Here's how the part is built. I have some questions about the finished solid (model axes, mm). A direction names the side the tool comes from. Coordinates: 2 decimals unless noted, no trailing zeros. Write each loop counter-clockwise with the first axis right and the second up, starting at its lowest first coordinate (ties: lowest second). Pieces come first, ordered by that corner, then holes. Notation, with made-up numbers: (58.5, 62.25) -> (102.5, 62.25) arc R12 cw to (102.5, 75.25) -> close; hole circle Ø1 at (54.5, 87.25). An arc over 180 degrees is marked (long way). Put each result on its own line as item: value. Start each with the question number.
Item 1: I need wall thicknesses on line 1 (Y direction, x = -3.5, z = 9.5); line 2 (X direction, y = 45.5, z = -1); line 3 (Y direction, x = -2, z = 5.25). Which ranges of each line are inside material? Lowest first, please. Write a range as [from, to].
Item 2: I want a section at B-B, the plane x = 0. List the corners of the cut face in (y, z) for me, then the cut area to 3 significant figures.
Item 3: I want a section at A-A, the plane y = 42. List the corners of the cut face in (x, z) for me, then the cut area to 3 significant figures.
Item 4: On a 3-axis mill with a long thin cutter (end or side, diameter ignored), from which of +Z, -Z, +X, -X, +Y, -Y can I reach the whole of each face in a straight line? I mean faces 1 (the face through (1.72, 9.09, 8.11)), 2 (the face through (-4.55, 31, -4)), 3 (the face through (4.492, 31, 5)), 4 (the face through (-4, 31, -5.11)). Say none if no direction works.
Item 5: For pin 1 (0.8 mm diameter, centred on x = -4, y = 32.5, fed in from -Z); pin 2 (0.6 mm diameter, centred on y = 52, z = 2.5, fed in from +X); pin 3 (6 mm diameter, centred on x = -3, y = 35.5, fed in from +Z), each with a flat end and sliding along its axis, tell me the tip position at first contact or that it passes through.
Item 6: I want a section at C-C, the plane y = 5.5. List the corners of the cut face in (x, z) for me, then the cut area to 3 significant figures.
Item 7: If we mould it in two halves opening along Y, with no side actions, what happens to faces 5 (the face through (0, 0, 1)), 6 (the face through (3.947, 31, 0)), 7 (the face through (-4, 31, 5.846)), 8 (the face through (0, 52.9, 0))? For each: released by +Y, released by -Y, zero draft, split by the parting line, or undercut.
Autodesk Inventor part; units mm, degrees
ref_plane "YZ Plane" through (0, 0, 0) normal (1, 0, 0) x (0, 1, 0)
ref_plane "XZ Plane" through (0, 0, 0) normal (0, 1, 0) x (-1, 0, 0)
ref_plane "XY Plane" through (0, 0, 0) normal (0, 0, 1) x (1, 0, 0)
sketch "草圖1" plane through (0, 0, 0) normal (0, 1, 0) x (-1, 0, 0)
  circle A0 centre (0, 0.3443) radius 12
  point P0 (0, 0)
  dimension "d0" = 24
extrude "擠出1" add sketch "草圖1" along normal blind 11
draft "面拔模1" angle 24 pull direction (0, 1, 0) faces at (-11.8446, 7.3333, -1.5807) fixed edges at (12, 0, 0.3443)
sketch "草圖2" plane through (0, 11, 0.3443) normal (0, 1, 0) x (1, 0, 0)
  line L0 (-4.5495, -3.8466) -> (-2.9152, -3.8466)
  line L1 (-2.9152, -3.8466) -> (-2.9152, -5.5016)
  line L2 (-2.9152, -5.5016) -> (-4.5495, -5.5016)
  line L3 (-4.5495, -5.5016) -> (-4.5495, -3.8466)
  circle A0 centre (0, 0) radius 7.1025
  line L4 (-4.5495, 5.4541) -> (-2.9152, 5.4541)
  line L5 (-2.9152, 5.4541) -> (-2.9152, 3.8283)
  line L6 (-2.9152, 3.8283) -> (-4.5495, 3.8283)
  line L7 (-4.5495, 3.8283) -> (-4.5495, 5.4541)
  line L8 (4.5495, 5.4541) -> (2.8978, 5.4541)
  line L9 (2.8978, 5.4541) -> (2.8978, 3.8283)
  line L10 (2.8978, 3.8283) -> (4.5495, 3.8283)
  line L11 (4.5495, 3.8283) -> (4.5495, 5.4541)
  line L12 (4.492, -5.5016) -> (2.862, -5.5016)
  line L13 (2.862, -5.5016) -> (2.862, -3.8466)
  line L14 (2.862, -3.8466) -> (4.492, -3.8466)
  line L15 (4.492, -3.8466) -> (4.492, -5.5016)
  line L16 (-3.9212, 3.8283) -> (-3.9212, -3.8466)
  line L17 (-2.9152, -5.0387) -> (2.862, -5.0387)
  line L18 (3.9473, -3.8466) -> (3.9473, 3.8283)
  line L19 (2.8978, 4.9975) -> (-2.9152, 4.9975)
  point P0 (0, 0.3443)
  dimension "d4" = 1.63
extrude "擠出2" add sketch "草圖2" along normal blind 40 contours L0 L1 L2 A0 L3 | L16 L6 L5 L19 L9 L10 L18 L14 L13 L17 L1 L0 | A0 L2 L3 | L6 L7 L4 L5 | L11 L10 L9 L8 | L12 L13 L14 L15
sketch "草圖3" plane through (0, 51, 0.3443) normal (0, 1, 0) x (1, 0, 0)
  circle A0 centre (0, 0) radius 12
  line L0 (-4.5956, 11.0851) -> (4.5888, 11.088)
  line L1 (4.5888, 11.088) -> (11.0851, 4.5956)
  line L2 (11.0851, 4.5956) -> (11.088, -4.5888)
  line L3 (11.088, -4.5888) -> (4.5956, -11.0851)
  line L4 (4.5956, -11.0851) -> (-4.5888, -11.088)
  line L5 (-4.5888, -11.088) -> (-11.0851, -4.5956)
  line L6 (-11.0851, -4.5956) -> (-11.088, 4.5888)
  line L7 (-11.088, 4.5888) -> (-4.5956, 11.0851)
extrude "擠出3" add sketch "草圖3" along normal blind 2 contours L2 L3 L4 L5 L6 L7 L0 L1
sketch "草圖4" plane through (0, 53, 0.3443) normal (0, 1, 0) x (1, 0, 0)
  line L0 (5, -5) -> (5, 5)
  line L1 (5, 5) -> (-5, 5)
  line L2 (-5, 5) -> (-5, -5)
  line L3 (-5, -5) -> (5, -5)
  line L4 (5, -5) -> (-5, 5) construction
  line L5 (5, 5) -> (-5, -5) construction
  point P0 (0, 0.3443)
  point P1 (0, 0)
  dimension "d9" = 10
  dimension "d10" = 10
extrude "擠出4" cut sketch "草圖4" against normal blind 0.1
properties part number "盤子上布丁"
Calculated:
1. line 1: y = [0, 4.94], [51, 53]
1. line 2: x = [-3.92, 3.95]
1. line 3: y = [0, 52.9]
2. outline: (0, -11.66) -> (11, -6.76) -> (11, -4.65) -> (51, -4.65) -> (51, -10.74) -> (53, -10.74) -> (53, -4.66) -> (52.9, -4.66) -> (52.9, 5.34) -> (53, 5.34) -> (53, 11.43) -> (51, 11.43) -> (51, 5.38) -> (11, 5.38) -> (11, 7.45) -> (0, 12.34) -> close
2. area: 655 mm2
3. outline: (-4.55, -5.11) -> (-2.92, -5.11) -> (-2.92, -4.65) -> (2.9, -4.65) -> (2.9, -5.11) -> (4.55, -5.11) -> (4.55, -3.48) -> (3.95, -3.48) -> (3.95, 4.19) -> (4.49, 4.19) -> (4.49, 5.85) -> (2.86, 5.85) -> (2.86, 5.38) -> (-2.92, 5.38) -> (-2.92, 5.85) -> (-4.55, 5.85) -> (-4.55, 4.19) -> (-3.92, 4.19) -> (-3.92, -3.48) -> (-4.55, -3.48) -> close
3. area: 84.8 mm2
4. face 1: none
4. face 2: +Z, -Z, -X
4. face 3: +Z, +X
4. face 4: -Z, +X, -X
5. pin 1: stops at z = -5.11
5. pin 2: stops at x = 11.09
5. pin 3: stops at z = 5.85
6. outline: circle Ø19.1 at (0, 0.34)
6. area: 287 mm2
7. face 5: released by -Y
7. face 6: undercut
7. face 7: undercut
7. face 8: released by +Y
